Could you check a few things on this model? Use its own coordinates, in mm. Face numbers are marked on the shaded views. A direction names the side the tool comes from. Coordinates: 2 decimals unless noted, no trailing zeros. Write each loop counter-clockwise with the first axis right and the second up, starting at its lowest first coordinate (ties: lowest second). Pieces come first, ordered by that corner, then holes. Notation, with made-up numbers: (37.5, 2) - (46.5, 2) arc R23 ccw to (46.5, 25) - close; hole circle Ø4 at (30.5, -4). An arc over 180 degrees is marked (long way). Answer as a JSON object with one key per item and string values. Group by question number.
1) If we section it at C-C (x = -8.75): Write out the boundary of the cut face in (y, z).
2) Will these pins go through, and if not, where does the flat tip stop? pin 1 Ø1.1 at (x, y) = (1, 1) entering from +Z; pin 2 Ø1 at (x, y) = (-4.5, 1.5) entering from -Z; pin 3 Ø1.5 at (y, z) = (1.5, -1.5) entering from +X.
3) If we section it at D-D (y = -2.75): Write out the boundary of the cut face in (x, z), plus the area to 3 significant figures.
4) If we section it at A-A (y = 0): Write out the boundary of the cut face in (x, z).
5) We'd pull the mould along Z, two halves only. Please class the marked faces 1 and 2: released by +Z, released by -Z, zero draft, split by the parting line, or undercut.
6) Please list where these lines run through material, in increasing order: line 1 along X through (y, z) = (3.25, -0.75); line 2 along Z through (x, y) = (0.25, -1.75); line 3 along Z through (x, y) = (0.5, -1.75).
7) On a 3-axis mill with a long thin cutter (end or side, diameter ignored), from which of +Z, -Z, +X, -X, +Y, -Y can I reach the whole of each face in a straight line? I mean the marked faces 3 and 4. Say none if no direction works.
```python
from build123d import *

# Parameters (mm, degrees)
SKETCH_1_R          = 4
EXTRUDE_1_DEPTH     = 0.3
SKETCH_2_R          = 2
EXTRUDE_3_DEPTH     = 10
SKETCH_6_R          = 3
EXTRUDE_4_DEPTH     = 0.1
DOME_1_FACE_RADIUS  = 3
DOME_1_HEIGHT       = 1
CUT_EXTRUDE_2_DEPTH = 3
CHAMFER_1_SIZE      = 0.5


with BuildPart() as part:
    # 草图1 → 凸台-拉伸1 (new body)
    with BuildSketch(Plane(origin=(0, 0, 0), x_dir=(0, 0, -1), z_dir=(1, 0, 0))):
        Circle(SKETCH_1_R)
    extrude(amount=EXTRUDE_1_DEPTH)

    # 草图2 → 凸台-拉伸3 (add)
    with BuildSketch(Plane.ZY):
        Circle(SKETCH_2_R)
    extrude(amount=EXTRUDE_3_DEPTH)

    # 草图6 → 凸台-拉伸4 (add)
    with BuildSketch(Plane(origin=(0.3, 0, 0), x_dir=(0, 0, -1), z_dir=(1, 0, 0))):
        Circle(SKETCH_6_R)
    extrude(amount=EXTRUDE_4_DEPTH)

    # 圆顶1: a dome of height H over a round flat face of radius A is a cap of a sphere of radius (A * A + H * H) / (2 * H)
    dome_1_r = (DOME_1_FACE_RADIUS * DOME_1_FACE_RADIUS + DOME_1_HEIGHT * DOME_1_HEIGHT) / (2 * DOME_1_HEIGHT)
    dome_1_base = Plane((0.4, 0, 0), z_dir=(1, 0, 0))
    with Locations(dome_1_base.offset(DOME_1_HEIGHT - dome_1_r)):
        dome_1_ball = Sphere(dome_1_r, mode=Mode.PRIVATE)
    add(split(dome_1_ball, bisect_by=dome_1_base, keep=Keep.TOP, mode=Mode.PRIVATE))

    # 草图5 → 切除-拉伸2 (cut)
    with BuildSketch(Plane(origin=(0, 0, 0), x_dir=(0, 0, -1), z_dir=(1, 0, 0))):
        Polygon((0.3, 0.3), (1.9, 0.3), (1.9, -0.3), (0.3, -0.3), (0.3, -1.9), (-0.3, -1.9), (-0.3, -0.3), (-1.9, -0.3), (-1.9, 0.3), (-0.3, 0.3), (-0.3, 1.9), (0.3, 1.9), align=None)
    extrude(amount=CUT_EXTRUDE_2_DEPTH, mode=Mode.SUBTRACT)

    # 倒角1
    chamfer_1_edges = [part.edges().sort_by_distance(p)[0] for p in [
        (-10, 0, -2),
    ]]
    chamfer(chamfer_1_edges, length=CHAMFER_1_SIZE)


solid = part.part
```
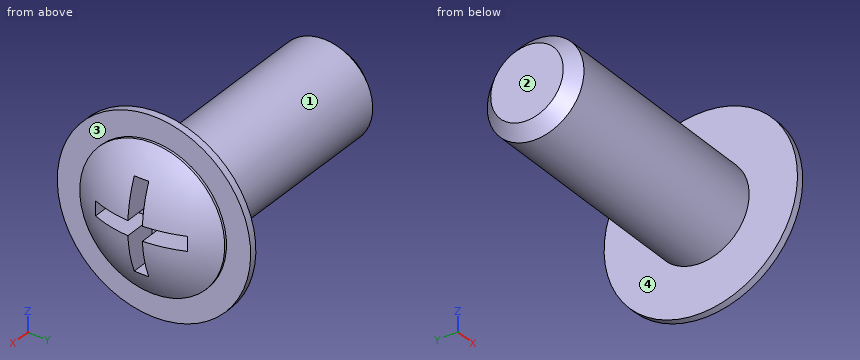
Here are the results:
{
 "1": {"outline": "circle Ø4 at (0, 0)"},
 "2": {"pin 1": "stops at z = 2.78", "pin 2": "stops at z = -1.73", "pin 3": "stops at x = 1.21"},
 "3": {"outline": "(0, -2.9) - (0.3, -2.9) - (0.3, -1.2) - (0.4, -1.2) arc R4.18 ccw to (0.4, 1.2) - (0.3, 1.2) - (0.3, 2.9) - (0, 2.9) - close", "area": "2.26 mm²"},
 "4": {"outline": "(-10, -1.5) - (-9.5, -2) - (0, -2) - (0, -4) - (0.3, -4) - (0.3, -3) - (0.4, -3) arc R5 ccw to (1.02, -1.9) - (0, -1.9) - (0, 1.9) - (1.02, 1.9) arc R5 ccw to (0.4, 3) - (0.3, 3) - (0.3, 4) - (0, 4) - (0, 2) - (-9.5, 2) - (-10, 1.5) - close"},
 "5": {"face 1": "split by the parting line", "face 2": "zero draft"},
 "6": {"line 1": "x = 0 to 0.3", "line 2": "z = -3.6 to -0.3, 0.3 to 3.6", "line 3": "z = -2.26 to -0.3, 0.3 to 2.26"},
 "7": {"face 3": "+X", "face 4": "-X"}
}
